Design review of the part built by this model. Coordinates are the model's own, in mm. Give positions to 0.01 mm unless a question says otherwise; leave off trailing zeros. Order: outer loops, then holes, each group sorted by start corner. A loop starts at its lowest first (then second) coordinate and runs counter-clockwise, first axis right, second up. Notation, with made-up numbers: (27.5, 80) -> (77.5, 80) arc R24 cw to (77.5, 111) -> close; hole circle Ø4 at (-30.5, -37). An arc over 180 degrees is marked (long way). One line per item, written item: value.
from build123d import *

# Parameters (mm, degrees)
SKETCH_1_R      = 3.5
SKETCH_1_R_2    = 1.25
EXTRUDE_1_DEPTH = 6.5
SKETCH_2_R      = 3.25
SKETCH_2_R_2    = 1.5
EXTRUDE_2_DEPTH = 7


with BuildPart() as part:
    # Эскиз1 → Бобышка-Вытянуть1 (new body)
    # profile 1 of 3: a face of its own
    with BuildSketch(Plane.XY):
        Circle(SKETCH_1_R)
        with Locations(Location((0, 0, 0), (0, 0, 180))):
            Circle(SKETCH_1_R_2, mode=Mode.SUBTRACT)
    # profile 2 of 3: a face of its own
    with BuildSketch(Plane.XY):
        with BuildLine():
            Line((3.5, 3.5), (0, 3.5))
            ThreePointArc((0, 3.5), (2.474873734, 2.474873734), (3.5, 0))
            Line((3.5, 0), (3.5, 3.5))
        make_face()
    # profile 3 of 3: a face of its own
    with BuildSketch(Plane.XY):
        with BuildLine():
            Line((3.5, -3.5), (3.5, 0))
            ThreePointArc((3.5, 0), (2.474873734, -2.474873734), (0, -3.5))
            Line((0, -3.5), (3.5, -3.5))
        make_face()
    extrude(amount=EXTRUDE_1_DEPTH)

    # Эскиз2 → Бобышка-Вытянуть2 (add)
    # profile 1 of 2: a face of its own
    with BuildSketch(Plane(origin=(0, 3.5, 0), x_dir=(1, 0, 0), z_dir=(0, 1, 0))):
        with BuildLine():
            ThreePointArc((7.5, -6.5), (4.25, -3.25), (7.5, 0))
            Line((7.5, 0), (3.5, 0))
            Line((3.5, 0), (3.5, -6.5))
            Line((3.5, -6.5), (7.5, -6.5))
        make_face()
    # profile 2 of 2: a face of its own
    with BuildSketch(Plane(origin=(0, 3.5, 0), x_dir=(1, 0, 0), z_dir=(0, 1, 0))):
        with Locations((7.5, -3.25)):
            Circle(SKETCH_2_R)
        with Locations(Location((7.5, -3.25, 0), (0, 0, 180))):
            Circle(SKETCH_2_R_2, mode=Mode.SUBTRACT)
    extrude(amount=-EXTRUDE_2_DEPTH)


solid = part.part
Item 1: Add section A-A on y = 0. Give the boundary of the cut face in (x, z), plus the area to 3 significant figures.
Returned:
outline: (-3.5, 0) -> (-1.25, 0) -> (-1.25, 6.5) -> (-3.5, 6.5) -> close; (1.25, 0) -> (7.5, 0) arc R3.25 ccw to (7.5, 6.5) -> (1.25, 6.5) -> close; hole circle Ø3 at (7.5, 3.25)
area: 64.8 mm²
Item 2: Add section C-C on x = 1. Give the boundary of the cut face in (y, z).
Returned:
outline: (-3.5, 0) -> (-0.75, 0) -> (-0.75, 6.5) -> (-3.5, 6.5) -> close; (0.75, 0) -> (3.5, 0) -> (3.5, 6.5) -> (0.75, 6.5) -> close
Item 3: Add section B-B on z = 3.25. Give the boundary of the cut face in (x, y), plus the area to 3 significant figures.
Returned:
outline: (0, -3.5) -> (6, -3.5) -> (6, 3.5) -> (0, 3.5) arc R3.5 ccw to start; (9, -3.5) -> (10.75, -3.5) -> (10.75, 3.5) -> (9, 3.5) -> close; hole circle Ø2.5 at (0, 0)
area: 68.6 mm²
Item 4: Add section D-D on z = 5.75. Give the boundary of the cut face in (x, y), plus the area to 3 significant figures.
Returned:
outline: (0, -3.5) -> (9.58, -3.5) -> (9.58, 3.5) -> (0, 3.5) arc R3.5 ccw to start; hole circle Ø2.5 at (0, 0)
area: 81.4 mm²
Item 5: Draft analysis for pull direction X (two halves, no side actions). For faces 1 (the cylindrical face through (-3.5, 0.1, 3.2)), 2 (the cylindrical face through (1.25, -0.05, 3.2)), 3 (the flat face through (2, 0, 0)), state which applies: pulls with the +X half, pulls with the -X half, needs draft (parallel to the pull), parting line crosses it, or undercut.
Returned:
face 1: pulls with the -X half
face 2: undercut
face 3: needs draft
Item 6: To check wall thickness, follow line 1 along Z through (x, y) = (7.5, 1.25); line 2 along X through (y, z) = (-3, 3.75); line 3 along Y through (x, z) = (0.25, 2.75). State the ranges of each line that lie inside material, in increasing order. Write a range as from..to.
Returned:
line 1: 0..1.75, 4.75..6.5
line 2: -1.8..6.09, 8.91..10.71
line 3: -3.5..-1.22, 1.22..3.5
